Can you work these out from the model? Positions are in its coordinate system, mm. A direction names the side the tool comes from. Give positions to 0.01 mm unless a question says otherwise; leave off trailing zeros. Loops run counter-clockwise (first coordinate to the right, second up) from the corner with the lowest first, then second, coordinate; pieces in that order, holes last. Notation, with made-up numbers: (5, -35) - (44, -35) arc R32 cw to (44, -9) - close; hole circle Ø2 at (25, -39). An arc over 180 degrees is marked (long way). Write item = value, one per line.
from build123d import *

# Parameters (mm, degrees)
SKETCH2_R           = 100
BOSS_EXTRUDE1_DEPTH = 30
SKETCH3_R           = 40
BOSS_EXTRUDE2_DEPTH = 150
CUT_EXTRUDE1_START  = -30
CUT_EXTRUDE1_DEPTH  = 30
BOSS_EXTRUDE6_DEPTH = 30
SKETCH6_R           = 20
BOSS_EXTRUDE7_DEPTH = 30


with BuildPart() as part:
    # Sketch2 → Boss-Extrude1 (new body)
    with BuildSketch(Plane.XY):
        Circle(SKETCH2_R)
    extrude(amount=BOSS_EXTRUDE1_DEPTH)

    # Sketch3 → Boss-Extrude2 (add)
    with BuildSketch(Plane.XY.offset(30)):
        Circle(SKETCH3_R)
    extrude(amount=BOSS_EXTRUDE2_DEPTH)

    # Sketch4 → Cut-Extrude1 (cut)
    with BuildSketch(Plane.XY.offset(180).offset(CUT_EXTRUDE1_START)):
        with BuildLine():
            Line((0, 40), (0, -40))
            ThreePointArc((0, -40), (40, 0), (0, 40))
        make_face()
    extrude(amount=CUT_EXTRUDE1_DEPTH, mode=Mode.SUBTRACT)

    # Sketch5 → Boss-Extrude6 (add)
    with BuildSketch(Plane.XY.offset(150)):
        with BuildLine():
            Line((100, 40), (0, 40))
            Line((0, 40), (0, -40))
            Line((0, -40), (100, -40))
            ThreePointArc((100, -40), (140, 0), (100, 40))
        make_face()
    extrude(amount=BOSS_EXTRUDE6_DEPTH)

    # Sketch6 → Boss-Extrude7 (add)
    with BuildSketch(Plane.XY.offset(180)):
        with Locations((100, 0)):
            Circle(SKETCH6_R)
    extrude(amount=BOSS_EXTRUDE7_DEPTH)


solid = part.part
Q1. Imagine slicing it at A-A, the plane y = 0. Write out the boundary of the cut face in (x, z), then the cut area to 3 significant figures.
Output:
outline = (-100, 0) - (100, 0) - (100, 30) - (40, 30) - (40, 150) - (140, 150) - (140, 180) - (120, 180) - (120, 210) - (80, 210) - (80, 180) - (-40, 180) - (-40, 30) - (-100, 30) - close
area = 22,200 mm2
Q2. For pin 1 (12 mm diameter, centred on x = 74.5, z = 164.5, fed in from +Y); pin 2 (8 mm diameter, centred on y = -39.5, z = 168.5, fed in from +X); pin 3 (24 mm diameter, centred on x = 68, y = -8.5, fed in from +Z), each with a flat end and sliding along its axis, tell me the tip position at first contact or that it passes through.
Output:
pin_1 = 40
pin_2 = 118.43
pin_3 = 180
Q3. I need wall thicknesses on L1, parallel to Z at x = -26, y = 67.5; L2, parallel to X at y = -1.5, z = 58; L3, parallel to Y at x = 89, z = 162. Which ranges of each line are inside material? Lowest first, please.
Output:
L1 = 0 to 30
L2 = -39.97 to 39.97
L3 = -40 to 40
Q4. Which directions (+Z, -Z, +X, -X, +Y, -Y) give clear straight access to the entire face, cutting with the end or side of a thin tool? Please do faces 1 (the cylindrical face through (95.38, 30.04, 14.79)), 2 (the flat face through (51, 40, 165)), 3 (the flat face through (-1, -43, 30)).
Output:
face_1 = -Z
face_2 = +Z, +X, -X, +Y
face_3 = none
Q5. Imagine slicing it at B-B, the plane x = 85. Write out the boundary of the cut face in (y, z).
Output:
outline = (-52.68, 0) - (52.68, 0) - (52.68, 30) - (-52.68, 30) - close; (-40, 150) - (40, 150) - (40, 180) - (13.23, 180) - (13.23, 210) - (-13.23, 210) - (-13.23, 180) - (-40, 180) - close
Q6. We'd pull the mould along Z, two halves only. Please class faces 4 (the flat face through (49, -40, 165)), 5 (the cylindrical face through (-39.96, 1.76, 103.95)), 6 (the flat face through (-1, 1, 0)): released by +Z, released by -Z, zero draft, split by the parting line, or undercut.
Output:
face_4 = zero draft
face_5 = undercut
face_6 = released by -Z
Q7. Imagine slicing it at C-C, the plane z = 72. Write out the boundary of the cut face in (x, y), then the cut area to 3 significant figures.
Output:
outline = circle Ø80 at (0, 0)
area = 5,030 mm2
Q8. Imagine slicing it at D-D, the plane x = 56.5. Write out the boundary of the cut face in (y, z), then the cut area to 3 significant figures.
Output:
outline = (-82.51, 0) - (82.51, 0) - (82.51, 30) - (-82.51, 30) - close; (-40, 150) - (40, 150) - (40, 180) - (-40, 180) - close
area = 7,350 mm2
